Geometry check sheet. Reference: the model listing, model coordinates, mm. Coordinates: 2 decimals unless noted, no trailing zeros. Write each loop counter-clockwise with the first axis right and the second up, starting at its lowest first coordinate (ties: lowest second). Pieces come first, ordered by that corner, then holes. Notation, with made-up numbers: (12.5, 18.25) -> (55.5, 18.25) arc R21 cw to (55.5, 57.25) -> close; hole circle Ø6 at (18.5, 37). An arc over 180 degrees is marked (long way). Answer in a Markdown table with one row per item. Add a question column.
Q1. Gauge pin test, flat ends, axial feed: P1, Ø3, axis at x = 7.78, z = 9.22, coming from the +Y side; P2, Ø2, axis at x = -7.112, z = 0, coming from the -Y side. Record the tip position at first contact, or that the pin passes through.
Q2. Section check C-C, the plane x = 1.25. Record the boundary of the cut face in (y, z), and give its area (3 significant figures).
Q3. Release check for a two-part mould opening along X. For faces 1 (the face through (0.534, 2.287, -5.413)), 2 (the face through (-3, 0, 0)), 3 (the face through (12.7, 3, 0)) record: pulls with the +X half, pulls with the -X half, needs draft (parallel to the pull), parting line crosses it, or undercut.
Q4. Thickness scan on line 1 (Z direction, x = 1, y = 2.55); line 2 (Z direction, x = 8.5, y = 2.9); line 3 (X direction, y = 2.6, z = 1). Record the ranges inside material, lowest first.
Q5. Section check A-A, the plane x = -2. Record the boundary of the cut face in (y, z), and give its area (3 significant figures).
Q6. Section check B-B, the plane y = 2. Count the separate pieces of the cut face and the enclosed holes in it, and give its area (3 significant figures).
```python
from build123d import *

# Parameters (mm, degrees)
SKETCH2_W                = 25.4
SKETCH2_H                = 38.1
BOSS_EXTRUDE1_DEPTH      = 5.08
CUT_EXTRUDE1_START       = -2.790735945
SKETCH7_R                = 2.4638
CUT_EXTRUDE1_DEPTH       = 11.685356434
CUT_EXTRUDE2_START       = -12.037410464
SKETCH16_R               = 2.4638
CUT_EXTRUDE2_DEPTH       = 14.163842911
M3_CLEARANCE_HOLE1_D     = 3.4
M3_CLEARANCE_HOLE1_DEPTH = 25.4
M3_CLEARANCE_HOLE1_TIP   = 1.021463052
M2_CLEARANCE_HOLE1_D     = 2.4
M2_CLEARANCE_HOLE1_DEPTH = 25.4
M2_CLEARANCE_HOLE1_TIP   = 0.721032743
M2_CLEARANCE_HOLE2_D     = 2.4
M2_CLEARANCE_HOLE2_DEPTH = 25.4
M2_CLEARANCE_HOLE2_TIP   = 0.721032743


with BuildPart() as part:
    # Sketch2 → Boss-Extrude1 (new body)
    with BuildSketch(Plane(origin=(0, 0, 0), x_dir=(1, 0, 0), z_dir=(0, 1, 0))):
        Rectangle(SKETCH2_W, SKETCH2_H)
    extrude(amount=BOSS_EXTRUDE1_DEPTH)

    # Sketch7 → Cut-Extrude1 (cut)
    with BuildSketch(Plane(origin=(12.7, 5.08, 4.3561), x_dir=(-1, 0, 0), z_dir=(0, -0.992546152, -0.121869343)).offset(CUT_EXTRUDE1_START)):
        with Locations((12.7, 1.016)):
            Circle(SKETCH7_R)
    cut_extrude1 = extrude(amount=CUT_EXTRUDE1_DEPTH, mode=Mode.SUBTRACT)

    # Sketch16 → Cut-Extrude2 (cut)
    with BuildSketch(Plane(origin=(12.7, 5.08, 13.0683), x_dir=(1, 0, 0), z_dir=(0, 0.982109046, 0.188313096)).offset(CUT_EXTRUDE2_START)):
        with Locations((-12.7, 3.048)):
            Circle(SKETCH16_R)
    cut_extrude2 = extrude(amount=CUT_EXTRUDE2_DEPTH, mode=Mode.SUBTRACT)

    # Mirror2: Cut-Extrude1, Cut-Extrude2 across plane
    add(cut_extrude1.mirror(Plane(origin=(0, 0, 0), x_dir=(1, 0, 0), z_dir=(0, 0, -1))), mode=Mode.SUBTRACT)
    add(cut_extrude2.mirror(Plane(origin=(0, 0, 0), x_dir=(1, 0, 0), z_dir=(0, 0, -1))), mode=Mode.SUBTRACT)

    # M3 Clearance Hole1
    with Locations(Plane(origin=(0, 5.08, 0), x_dir=(1, 0, 0), z_dir=(0, 1, 0))):
        with Locations((7.112, 0), (-7.112, 0)):
            Hole(M3_CLEARANCE_HOLE1_D / 2, depth=M3_CLEARANCE_HOLE1_DEPTH)
            with Locations((0, 0, -(M3_CLEARANCE_HOLE1_DEPTH + M3_CLEARANCE_HOLE1_TIP / 2))):  # 118° drill point
                Cone(0, M3_CLEARANCE_HOLE1_D / 2, M3_CLEARANCE_HOLE1_TIP, mode=Mode.SUBTRACT)

    # M2 Clearance Hole1
    with Locations(Plane(origin=(0, 5.08, 0), x_dir=(1, 0, 0), z_dir=(0, 1, 0))):
        with Locations((-7.573257477, -10.205203742), (-7.573257477, 10.942943937)):
            Hole(M2_CLEARANCE_HOLE1_D / 2, depth=M2_CLEARANCE_HOLE1_DEPTH)
            with Locations((0, 0, -(M2_CLEARANCE_HOLE1_DEPTH + M2_CLEARANCE_HOLE1_TIP / 2))):  # 118° drill point
                Cone(0, M2_CLEARANCE_HOLE1_D / 2, M2_CLEARANCE_HOLE1_TIP, mode=Mode.SUBTRACT)

    # M2 Clearance Hole2
    with Locations(Plane(origin=(0, 5.08, 0), x_dir=(1, 0, 0), z_dir=(0, 1, 0))):
        with Locations((7.779654049, -9.22186476), (7.779654049, 10.457647724)):
            Hole(M2_CLEARANCE_HOLE2_D / 2, depth=M2_CLEARANCE_HOLE2_DEPTH)
            with Locations((0, 0, -(M2_CLEARANCE_HOLE2_DEPTH + M2_CLEARANCE_HOLE2_TIP / 2))):  # 118° drill point
                Cone(0, M2_CLEARANCE_HOLE2_D / 2, M2_CLEARANCE_HOLE2_TIP, mode=Mode.SUBTRACT)


solid = part.part
```
Calculated:
| question | item | result |
|---|---|---|
| 1 | P1 | stops at y = 5.08 |
| 1 | P2 | passes through |
| 2 | outline | (0, -19.05) -> (5.08, -19.05) -> (5.08, -12.13) -> (0, -11.15) -> close; (0, -6.83) -> (5.08, -7.8) -> (5.08, -5.47) -> (0, -4.85) -> close; (0, -0.57) -> (5.08, -1.19) -> (5.08, 1.19) -> (0, 0.57) -> close; (0, 4.85) -> (5.08, 5.47) -> (5.08, 7.8) -> (0, 6.83) -> close; (0, 11.15) -> (5.08, 12.13) -> (5.08, 19.05) -> (0, 19.05) -> close |
| 2 | area | 106 mm² |
| 3 | face 1 | undercut |
| 3 | face 2 | needs draft |
| 3 | face 3 | pulls with the +X half |
| 4 | line 1 | z = -19.05 to -11.77, -7.19 to -5.29, -0.75 to 0.75, 5.29 to 7.19, 11.77 to 19.05 |
| 4 | line 2 | z = -19.05 to -11.42, -9.5 to -0.98, 0.98 to 8.26, 10.18 to 19.05 |
| 4 | line 3 | x = -12.7 to -8.49, -5.74 to -1.42, 1.42 to 5.74, 8.49 to 12.7 |
| 5 | outline | (0, -19.05) -> (5.08, -19.05) -> (5.08, -11.43) -> (0, -10.46) -> close; (0, -7.53) -> (5.08, -8.5) -> (5.08, -4.78) -> (0, -4.16) -> close; (0, -1.26) -> (5.08, -1.88) -> (5.08, 1.88) -> (0, 1.26) -> close; (0, 4.16) -> (5.08, 4.78) -> (5.08, 8.5) -> (0, 7.53) -> close; (0, 10.46) -> (5.08, 11.43) -> (5.08, 19.05) -> (0, 19.05) -> close |
| 5 | area | 134 mm² |
| 6 | separate pieces | 1 |
| 6 | enclosed holes | 10 |
| 6 | area | 854 mm² |
